For this review, take the finished solid that the model builds, in its own axes (mm). Face numbers are marked on the shaded views. A direction names the side the tool comes from. Round coordinates to 2 decimals unless told otherwise and drop trailing zeros. Order: outer loops, then holes, each group sorted by start corner. A loop starts at its lowest first (then second) coordinate and runs counter-clockwise, first axis right, second up. Notation, with made-up numbers: (25.25, -24.5) -> (58.25, -24.5) arc R26 cw to (58.25, -4.5) -> close; hole circle Ø1 at (31.25, -13.75). An arc over 180 degrees is marked (long way). Use a Markdown table: item, result. Add a question column.
1) Consider section C-C (x = 14.5). State the section outline as (y, z) points.
2) Clearance check with flat-ended pins moving along their axes: P1, Ø2, axis at x = 25.5, y = -17, coming from the -Z side; P2, Ø4, axis at x = 43.5, z = 16, coming from the -Y side; P3, Ø2, axis at x = 27.5, y = -18, coming from the +Z side. State where each tip first meets the part, or that it passes through.
3) Consider section D-D (x = 45.5). State the section outline as (y, z) points.
4) Machinability: for the marked faces 1 and 2, which of the approach directions +Z, -Z, +X, -X, +Y, -Y give a long, thin tool a straight path to every point of the face, cutting with its end or side? Answer none if there is none.
5) Wall thickness on line 1 along Z through (x, y) = (25.4, -7.5); line 2 along Z through (x, y) = (25.4, -18.5): over which ranges is each line inside the solid? List them lowest first. Write a range as [from, to].
6) Consider section A-A (y = -11). State the section outline as (x, z) points.
7) Consider section B-B (z = 24.5). State the section outline as (x, y) points.
```python
from build123d import *

# Parameters (mm, degrees)
F0_W     = 57.15
F0_H     = 44.45
F1_DEPTH = 25.4
F3_DEPTH = 25.401
F5_DEPTH = 12.7


with BuildPart() as f1:
    # F0 (on Front) → F1 (new body)
    with BuildSketch(Plane.XZ):
        with Locations((28.575, 22.225)):
            Rectangle(F0_W, F0_H)
    extrude(amount=F1_DEPTH)

    # F2 (on face) → F3 (cut, through all)
    with BuildSketch(Plane.XZ.offset(25.4)):
        with BuildLine():
            ThreePointArc((25.4, 38.1), (16.4197438789, 16.4197438789), (38.1, 25.4))
            ThreePointArc((38.1, 25.4), (34.3802561211, 34.3802561211), (25.4, 38.1))
        make_face()
    extrude(amount=-F3_DEPTH, mode=Mode.SUBTRACT)

    # F4 (on face) → F5 (cut)
    with BuildSketch(Plane.XZ.offset(25.4)):
        with BuildLine():
            Line((57.15, 44.45), (18.9351793379, 44.45))
            Line((18.9351793379, 44.45), (22.225, 37.6967221242))
            ThreePointArc((22.225, 37.6967221242), (33.1771299333, 35.440231571), (38.1, 25.4))
            ThreePointArc((38.1, 25.4), (36.7085708258, 19.6201880759), (32.8391770271, 15.1068641727))
            Line((32.8391770271, 15.1068641727), (44.45, 0))
            Line((44.45, 0), (57.15, 0))
            Line((57.15, 0), (57.15, 44.45))
        make_face()
    extrude(amount=-F5_DEPTH, mode=Mode.SUBTRACT)


solid = f1.part
```
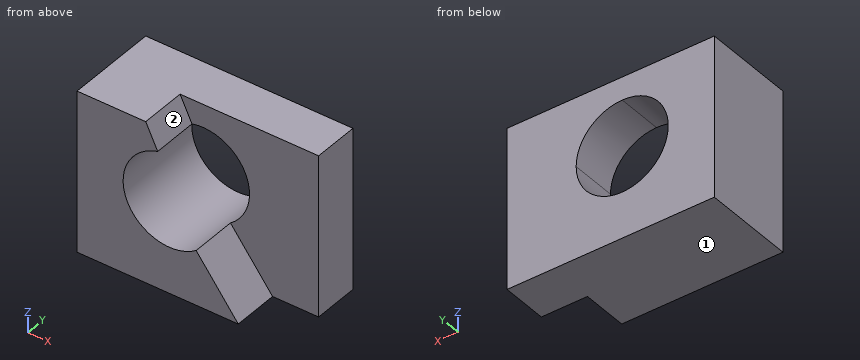
Results list:
| question | item | result |
|---|---|---|
| 1 | outline | (-25.4, 0) -> (0, 0) -> (0, 18.88) -> (-25.4, 18.88) -> close; (-25.4, 31.92) -> (0, 31.92) -> (0, 44.45) -> (-25.4, 44.45) -> close |
| 2 | P1 | z = 0 |
| 2 | P2 | y = -12.7 |
| 2 | P3 | z = 13.08 |
| 3 | outline | (-12.7, 0) -> (0, 0) -> (0, 44.45) -> (-12.7, 44.45) -> close |
| 4 | face 1 | -Z, +X, -X, +Y, -Y |
| 4 | face 2 | +Z, +X, -Y |
| 5 | line 1 | [0, 12.7], [38.1, 44.45] |
| 5 | line 2 | [0, 12.7] |
| 6 | outline | (0, 0) -> (57.15, 0) -> (57.15, 44.45) -> (0, 44.45) -> close; hole circle Ø25.4 at (25.4, 25.4) |
| 7 | outline | (0, -25.4) -> (12.73, -25.4) -> (12.73, 0) -> (0, 0) -> close; (38.07, -12.7) -> (57.15, -12.7) -> (57.15, 0) -> (38.07, 0) -> close |
